```python
from build123d import *

# Parameters (mm, degrees)
SKETCH1_W                        = 44.45
SKETCH1_H                        = 44.45
SKETCH1_R                        = 11.176
BOSS_EXTRUDE1_DEPTH              = 3.175
F_10_0_1935_DIAMETER_HOLE1_D     = 4.9149
F_10_0_1935_DIAMETER_HOLE1_DEPTH = 3.175
CSK_FOR_M3_SFHCS1_AT_2_COUNT     = 2
CSK_FOR_M3_SFHCS1_AT_2_PITCH     = 16
CSK_FOR_M3_SFHCS1_AT_3_COUNT     = 2
CSK_FOR_M3_SFHCS1_AT_3_PITCH     = 27.712812921
CSK_FOR_M3_SFHCS1_AT_4_COUNT     = 2
CSK_FOR_M3_SFHCS1_AT_4_PITCH     = 32
CSK_FOR_M3_SFHCS1_AT_5_COUNT     = 2
CSK_FOR_M3_SFHCS1_AT_5_PITCH     = 27.712812921
CSK_FOR_M3_SFHCS1_AT_6_COUNT     = 2
CSK_FOR_M3_SFHCS1_AT_6_PITCH     = 16
FILLET1_R                        = 3.175


with BuildPart() as part:
    # Sketch1 → Boss-Extrude1 (new body)
    with BuildSketch(Plane(origin=(0, 0, 0), x_dir=(0, 0, -1), z_dir=(1, 0, 0))):
        Rectangle(SKETCH1_W, SKETCH1_H)
        Circle(SKETCH1_R, mode=Mode.SUBTRACT)
    extrude(amount=BOSS_EXTRUDE1_DEPTH)

    # #10 (0.1935) Diameter Hole1
    with Locations(Plane(origin=(3.175, 0, 0), x_dir=(0, 0, -1), z_dir=(1, 0, 0))):
        with Locations((-17.4625, 17.4625), (17.4625, 17.4625), (17.4625, -17.4625), (-17.4625, -17.4625)):
            Hole(F_10_0_1935_DIAMETER_HOLE1_D / 2, depth=F_10_0_1935_DIAMETER_HOLE1_DEPTH)

    # Sketch6 → CSK for M3 SFHCS1 (revolve, cut)
    with BuildSketch(Plane(origin=(3.175, 8, 13.856406461), x_dir=(0, 0, -1), z_dir=(0, 1, 0))):
        Polygon((0, 0), (0, 3.175), (1.7, 3.175), (1.7, 1.66), (3.36, 0), align=None)
    csk_for_m3_sfhcs1 = revolve(axis=Axis((9.525, 8, 13.856406461), (-1, 0, 0)), mode=Mode.SUBTRACT)

    # CSK for M3 SFHCS1 at 2: CSK for M3 SFHCS1 ×2
    with Locations(*[Vector(0, 0.5, -0.866025404) * (i * CSK_FOR_M3_SFHCS1_AT_2_PITCH) for i in range(1, CSK_FOR_M3_SFHCS1_AT_2_COUNT)]):
        add(csk_for_m3_sfhcs1, mode=Mode.SUBTRACT)

    # CSK for M3 SFHCS1 at 3: CSK for M3 SFHCS1 ×2
    with Locations(*[(0, 0, -i * CSK_FOR_M3_SFHCS1_AT_3_PITCH) for i in range(1, CSK_FOR_M3_SFHCS1_AT_3_COUNT)]):
        add(csk_for_m3_sfhcs1, mode=Mode.SUBTRACT)

    # CSK for M3 SFHCS1 at 4: CSK for M3 SFHCS1 ×2
    with Locations(*[Vector(0, -0.5, -0.866025404) * (i * CSK_FOR_M3_SFHCS1_AT_4_PITCH) for i in range(1, CSK_FOR_M3_SFHCS1_AT_4_COUNT)]):
        add(csk_for_m3_sfhcs1, mode=Mode.SUBTRACT)

    # CSK for M3 SFHCS1 at 5: CSK for M3 SFHCS1 ×2
    with Locations(*[Vector(0, -0.866025404, -0.5) * (i * CSK_FOR_M3_SFHCS1_AT_5_PITCH) for i in range(1, CSK_FOR_M3_SFHCS1_AT_5_COUNT)]):
        add(csk_for_m3_sfhcs1, mode=Mode.SUBTRACT)

    # CSK for M3 SFHCS1 at 6: CSK for M3 SFHCS1 ×2
    with Locations(*[(0, -i * CSK_FOR_M3_SFHCS1_AT_6_PITCH, 0) for i in range(1, CSK_FOR_M3_SFHCS1_AT_6_COUNT)]):
        add(csk_for_m3_sfhcs1, mode=Mode.SUBTRACT)

    # Fillet1
    fillet1_edges = [part.edges().sort_by_distance(p)[0] for p in [
        (1.5875, 22.225, 22.225),
        (1.5875, 22.225, -22.225),
        (1.5875, -22.225, -22.225),
        (1.5875, -22.225, 22.225),
    ]]
    fillet(fillet1_edges, radius=FILLET1_R)


solid = part.part
```
Model file for the job. Use its own axes, mm. Give positions to 0.01 mm unless a question says otherwise; leave off trailing zeros. Write each loop counter-clockwise with the first axis right and the second up, starting at its lowest first coordinate (ties: lowest second). Pieces come first, ordered by that corner, then holes. Notation, with made-up numbers: (-12.75, -36) -> (1.25, -36) arc R4 ccw to (1.25, -31) -> close; hole circle Ø11 at (-1, -15). An arc over 180 degrees is marked (long way). Use CSV: the item, a comma, the result in double quotes. Start each with the question number.
1) Cut at D-D on z = 6. List the corners of the cut face in (x, y) (3 decimals).
2) Cut at C-C on y = 16. List the corners of the cut face in (x, z) (3 decimals).
3) Two-plate mould, pull along Y, no slides. Class faces 1 (the flat face through (3.175, 5.3, 10.2)), 2 (the flat face through (2, 22.225, 0)), 3 (the cylindrical face through (1.57, -19.64, 18.6)): released by +Y, released by -Y, zero draft, split by the parting line, or undercut.
4) Drill centre lines: L1, parallel to Y at x = 0.25, z = -14 (3 decimals); L2, parallel to Z at x = 0.35, y = 0.5 (3 decimals); L3, parallel to Z at x = 0.2, y = 16.5 (3 decimals). Where is each one in solid material? Low to high.
5) Cut at A-A on y = 0. List the corners of the cut face in (x, z) (3 decimals), plus the area to 3 significant figures.
6) Cut at B-B on z = 0. List the corners of the cut face in (x, y) (3 decimals), plus the area to 3 significant figures.
7) Pin check, flat tips, straight feed: P1, Ø5.5, axis at y = -8, z = 13.86, coming from the +X side; P2, Ø10, axis at y = 3.5, z = -3.5, coming from the +X side. Stop position of each tip, or through.
Final values:
1,outline,"(0, -22.225) -> (3.175, -22.225) -> (3.175, -9.429) -> (0, -9.429) -> close; (0, 9.429) -> (3.175, 9.429) -> (3.175, 22.225) -> (0, 22.225) -> close"
2,outline,"(0, -22.225) -> (3.175, -22.225) -> (3.175, -19.437) -> (0, -19.437) -> close; (0, -15.488) -> (3.175, -15.488) -> (3.175, -3.36) -> (1.515, -1.7) -> (0, -1.7) -> close; (0, 1.7) -> (1.515, 1.7) -> (3.175, 3.36) -> (3.175, 15.488) -> (0, 15.488) -> close; (0, 19.437) -> (3.175, 19.437) -> (3.175, 22.225) -> (0, 22.225) -> close"
3,face 1,"zero draft"
3,face 2,"released by +Y"
3,face 3,"undercut"
4,L1,"y = -22.225 to -9.694, -6.306 to 6.306, 9.694 to 22.225"
4,L2,"z = -22.225 to -11.165, 11.165 to 22.225"
4,L3,"z = -22.225 to -19.724, -15.201 to -1.625, 1.625 to 15.201, 19.724 to 22.225"
5,outline,"(0, -22.225) -> (3.175, -22.225) -> (3.175, -11.176) -> (0, -11.176) -> close; (0, 11.176) -> (3.175, 11.176) -> (3.175, 22.225) -> (0, 22.225) -> close"
5,area,"70.2 mm2"
6,outline,"(0, -22.225) -> (3.175, -22.225) -> (3.175, -19.36) -> (1.515, -17.7) -> (0, -17.7) -> close; (0, -14.3) -> (1.515, -14.3) -> (3.175, -12.64) -> (3.175, -11.176) -> (0, -11.176) -> close; (0, 11.176) -> (3.175, 11.176) -> (3.175, 12.64) -> (1.515, 14.3) -> (0, 14.3) -> close; (0, 17.7) -> (1.515, 17.7) -> (3.175, 19.36) -> (3.175, 22.225) -> (0, 22.225) -> close"
6,area,"43.1 mm2"
7,P1,"stops at x = 2.57"
7,P2,"passes through"
